Read the model definition and answer for the solid it produces. Units are mm, in the model's axes. A direction names the side the tool comes from. Give positions to 0.01 mm unless a question says otherwise; leave off trailing zeros. Order: outer loops, then holes, each group sorted by start corner. A loop starts at its lowest first (then second) coordinate and runs counter-clockwise, first axis right, second up. Notation, with made-up numbers: (24, 4) - (62, 4) arc R30 cw to (62, 35) - close; hole circle Ø11 at (7.5, 47.5). An arc over 180 degrees is marked (long way). Answer as CSV lines item,"result". Start each with the question number.
from build123d import *

# Parameters (mm, degrees)
SALIENTE_EXTRUIR1_DEPTH = 28
CROQUIS2_W              = 18
CROQUIS2_H              = 8
CORTAR_EXTRUIR1_DEPTH   = 99


with BuildPart() as part:
    # Croquis1 → Saliente-Extruir1 (new body)
    with BuildSketch(Plane.XY):
        Polygon((-20, 35), (20, 35), (31, -35), (42, -35), (42, -49), (-42, -49), (-42, -35), (-31, -35), align=None)
    extrude(amount=-SALIENTE_EXTRUIR1_DEPTH)

    # Croquis2 → Cortar-Extruir1 (cut, through all)
    with BuildSketch(Plane(origin=(0, 35, 0), x_dir=(1, 0, 0), z_dir=(0, 1, 0))):
        with Locations((0, 4)):
            Rectangle(CROQUIS2_W, CROQUIS2_H)
        with Locations((0, 24)):
            Rectangle(CROQUIS2_W, CROQUIS2_H)
    extrude(amount=-CORTAR_EXTRUIR1_DEPTH, mode=Mode.SUBTRACT)


solid = part.part
(1) Which of the six approach directions +Z, -Z, +X, -X, +Y, -Y give full straight-line access (tool end or side, diameter ignored) to faces 1 (the flat face through (42, -42, -14)), 2 (the flat face through (9, -6, -24)), 3 (the flat face through (-37, -35, -14)), 4 (the flat face through (36, -35, -14)), 5 (the flat face through (-9, -6, -4))?
(2) Section C-C, the plane y = 13 is taken. Write down the section's boundary in (x, z).
(3) Section B-B, the plane z = -23.5 is taken. Write down the section's boundary in (x, y), and give its area (3 significant figures).
(4) Section D-D, the plane x = 2.5 is taken. Write down the section's boundary in (y, z), and give its area (3 significant figures).
(5) Flat-ended cylindrical pins translate along their axes: pin 1 Ø9 at (x, z) = (37.5, -13) entering from +Y; pin 2 Ø2.5 at (y, z) = (-19.5, -5.5) entering from +X; pin 3 Ø5 at (y, z) = (-31, -10) entering from +X. Find the tip coordinate at first contact, or state that the pin passes through.
(6) Section A-A, the plane z = -14 is taken. Write down the section's boundary in (x, y).
(7) Determine the mould class of faces 6 (the flat face through (0, -6, -8)), 7 (the flat face through (-18, -16, -28)), 8 (the flat face through (-25.577, -0.49, -13.804)), 9 (the flat face through (25.423, 0.49, -13.804)) for opening direction X: released by +X, released by -X, zero draft, split by the parting line, or undercut.
(8) Straight lines are drawn through the part: line 1 (X direction, y = -10, z = -22.5); line 2 (Z direction, x = 5, y = 27); line 3 (X direction, y = 15, z = -6.5). For each, find the intervals that lie inside material, in ascending order. Write a range as [from, to].
Checks:
1,face 1,"+Z, -Z, +X, +Y, -Y"
1,face 2,"-Z, +Y, -Y"
1,face 3,"+Z, -Z, -X, +Y"
1,face 4,"+Z, -Z, +X, +Y"
1,face 5,"+Z, +Y, -Y"
2,outline,"(-23.46, -28) - (-9, -28) - (-9, -20) - (9, -20) - (9, -28) - (23.46, -28) - (23.46, 0) - (9, 0) - (9, -8) - (-9, -8) - (-9, 0) - (-23.46, 0) - close"
3,outline,"(-42, -49) - (-9, -49) - (-9, 35) - (-20, 35) - (-31, -35) - (-42, -35) - close; (9, -49) - (42, -49) - (42, -35) - (31, -35) - (20, 35) - (9, 35) - close"
3,area,"3,230 mm²"
4,outline,"(-49, -20) - (35, -20) - (35, -8) - (-49, -8) - close"
4,area,"1,010 mm²"
5,pin 1,"stops at y = -35"
5,pin 2,"stops at x = 28.76"
5,pin 3,"stops at x = 30.76"
6,outline,"(-42, -49) - (42, -49) - (42, -35) - (31, -35) - (20, 35) - (-20, 35) - (-31, -35) - (-42, -35) - close"
7,face 6,"undercut"
7,face 7,"zero draft"
7,face 8,"released by -X"
7,face 9,"released by +X"
8,line 1,"x = [-27.07, -9], [9, 27.07]"
8,line 2,"z = [-20, -8]"
8,line 3,"x = [-23.14, -9], [9, 23.14]"
